Job drawing, mm, ordinate dimensions from the low corner. One solid piece. Round coordinates to 2 decimals unless told otherwise and drop trailing zeros. Loops run counter-clockwise (first coordinate to the right, second up) from the corner with the lowest first, then second, coordinate; pieces in that order, holes last.
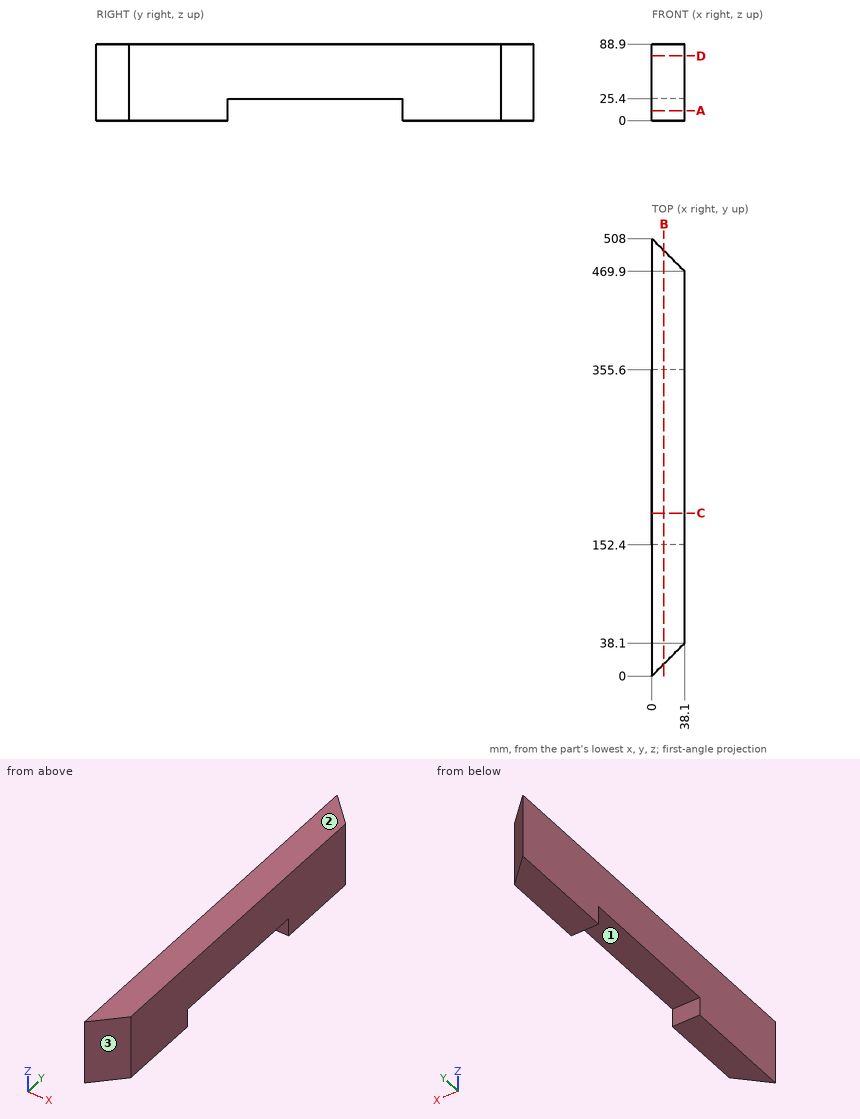
Item 1: Cut at C-C, the plane y = 189. Give the cut face in (x, z).
Answers follow:
outline: (0, 25.4) - (38.1, 25.4) - (38.1, 88.9) - (0, 88.9) - close
Item 2: Probe line 1 (Z direction, x = 17.5, y = 276.5); line 2 (Y direction, x = 30.5, z = 22.5); line 3 (Y direction, x = 23.5, z = 20). List the from-to ranges inside material, lowest first.
Answers follow:
line 1: z = 25.4 to 88.9
line 2: y = 30.5 to 152.4, 355.6 to 477.5
line 3: y = 23.5 to 152.4, 355.6 to 484.5
Item 3: Cut at D-D, the plane z = 75. Give the cut face in (x, y).
Answers follow:
outline: (0, 0) - (38.1, 38.1) - (38.1, 469.9) - (0, 508) - close
Item 4: Flat gauge pins, fed straight in: P1, Ø8, axis at x = 10.5, y = 304.5, coming from the -Z side; P2, Ø20.5, axis at x = 13.5, z = 8.5, coming from the -Y side; P3, Ø12, axis at x = 8.5, z = 38, coming from the -Y side. Where does each tip first touch, or does it go through?
Answers follow:
P1: stops at z = 25.4
P2: stops at y = 3.25
P3: stops at y = 2.5
Item 5: Cut at A-A, the plane z = 11.5. Give the cut face in (x, y), plus the area to 3 significant figures.
Answers follow:
outline: (0, 0) - (38.1, 38.1) - (38.1, 152.4) - (0, 152.4) - close; (0, 355.6) - (38.1, 355.6) - (38.1, 469.9) - (0, 508) - close
area: 10,200 mm2
Item 6: Two-plate mould, pull along Y, no slides. Class the marked faces 1, 2 and 3: released by +Y, released by -Y, zero draft, split by the parting line, or undercut.
Answers follow:
face 1: undercut
face 2: zero draft
face 3: released by -Y
Item 7: Cut at B-B, the plane x = 14. Give the cut face in (y, z).
Answers follow:
outline: (14, 0) - (152.4, 0) - (152.4, 25.4) - (355.6, 25.4) - (355.6, 0) - (494, 0) - (494, 88.9) - (14, 88.9) - close
